from build123d import *

# Parameters (mm, degrees)
F0_W     = 38.1
F0_H     = 38.1
F1_DEPTH = 38.1
F4_DEPTH = 38.1


with BuildPart() as f1:
    # F0 (on Front) → F1 (new body)
    with BuildSketch(Plane.XZ):
        with Locations((19.05, 19.05)):
            Rectangle(F0_W, F0_H)
    extrude(amount=F1_DEPTH)

    # F3 (on face) → F4 (cut)
    with BuildSketch(Plane.XZ.offset(38.1)):
        Polygon((31.757813, 38.1), (6.35, 38.1), (11.43, 14.032523), (16.517813, 28.575), (21.597813, 28.575), (26.677813, 15.509631), align=None)
        Polygon((6.35, 0), (0, 38.1), (0, 0), align=None)
        Polygon((19.05, 15.875), (12.7, 0), (25.4, 0), align=None)
        Polygon((38.1, 0), (38.1, 38.1), (31.75, 0), align=None)
    extrude(amount=-F4_DEPTH, mode=Mode.SUBTRACT)


solid = f1.part
Design review of the part built by this model. Coordinates are the model's own, in mm. A direction names the side the tool comes from. Coordinates: 2 decimals unless noted, no trailing zeros. Loops run counter-clockwise (first coordinate to the right, second up) from the corner with the lowest first, then second, coordinate; pieces in that order, holes last. Notation, with made-up numbers: (6, 27.5) - (62, 27.5) arc R19 ccw to (62, 38.5) - close; hole circle Ø10 at (22.5, 20.5). An arc over 180 degrees is marked (long way). Use CSV: the item, a comma, the result in double quotes. Start each with the question number.
1. Add section A-A on z = 8. Give the boundary of the cut face in (x, y).
2. Clearance check with flat-ended pins moving along their axes: pin 1 (2 mm diameter, centred on y = -18.5, z = 4, fed in from -X); pin 2 (1.5 mm diameter, centred on y = -24.5, z = 16, fed in from -X); pin 3 (1 mm diameter, centred on y = -17.5, z = 29, fed in from -X). State where each tip first meets the part, or that it passes through.
3. Add section C-C on y = -30.5. Give the boundary of the cut face in (x, z) (3 decimals), plus the area to 3 significant figures.
4. Mouldability with a two-part tool opening along X and no side actions: class faces 1 (the flat face through (24.102, -19.317, 22.134)), 2 (the flat face through (34.97, -19.32, 19.32)), 3 (the flat face through (35, -19, 38.1)), 4 (the flat face through (8.854, -19.317, 26.235)) as released by +X, released by -X, zero draft, split by the parting line, or undercut.
5. Add section D-D on x = 18. Give the boundary of the cut face in (y, z) (3 decimals), plus the area to 3 significant figures.
6. Add section B-B on z = 17.5. Give the boundary of the cut face in (x, y).
7. To check wall thickness, follow probe 1 along X at (y, z) = (-6.5, 18.5); probe 2 along X at (y, z) = (-24, 27); probe 3 along X at (y, z) = (-22.5, 32). State the ranges of each line that lie inside material, in increasing order.
8. For faces 5 (the flat face through (13.938, -19.317, 21.202)), 6 (the flat face through (19, 0, 19)), 7 (the flat face through (15.9, -19.3, 8)), list the 3-axis set-ups (+Z, -Z, +X, -X, +Y, -Y) from which the entire face can be reached by the end or side of a thin tool; tool diameter is ignored.
Resolved:
1,outline,"(5.02, -38.1) - (15.9, -38.1) - (15.9, 0) - (5.02, 0) - close; (22.2, -38.1) - (33.08, -38.1) - (33.08, 0) - (22.2, 0) - close"
2,pin 1,"x = 5.52"
2,pin 2,"x = 3.56"
2,pin 3,"x = 1.43"
3,outline,"(0, 38.1) - (6.35, 0) - (12.7, 0) - (19.05, 15.875) - (25.4, 0) - (31.75, 0) - (38.1, 38.1) - (31.758, 38.1) - (26.678, 15.51) - (21.598, 28.575) - (16.518, 28.575) - (11.43, 14.033) - (6.35, 38.1) - close"
3,area,"775 mm2"
4,face 1,"undercut"
4,face 2,"released by +X"
4,face 3,"zero draft"
4,face 4,"undercut"
5,outline,"(-38.1, 13.25) - (0, 13.25) - (0, 28.575) - (-38.1, 28.575) - close"
5,area,"584 mm2"
6,outline,"(3.43, -38.1) - (10.7, -38.1) - (10.7, 0) - (3.43, 0) - close; (12.64, -38.1) - (25.9, -38.1) - (25.9, 0) - (12.64, 0) - close; (27.13, -38.1) - (34.67, -38.1) - (34.67, 0) - (27.13, 0) - close"
7,probe 1,"3.27 to 10.49, 12.99 to 25.52, 27.35 to 34.83"
7,probe 2,"1.85 to 8.69, 15.97 to 22.21, 29.26 to 36.25"
7,probe 3,"1.02 to 7.64, 30.39 to 37.08"
8,face 5,"+Z, +Y, -Y"
8,face 6,"+Z, -Z, +X, -X, +Y"
8,face 7,"-Z, +Y, -Y"
